Here's the drawing with two shaded views (mm, measured from the low corner). I have some questions. A direction names the side the tool comes from. Give positions to 0.01 mm unless a question says otherwise; leave off trailing zeros. Order: outer loops, then holes, each group sorted by start corner. A loop starts at its lowest first (then second) coordinate and runs counter-clockwise, first axis right, second up. Notation, with made-up numbers: M 34,63.25 L 73,63.25 A29 cw 73,84.25 Z; hole C 79.25,70 d6. An arc over 180 degrees is marked long. Use a Markdown table: item, result. Add a question column.
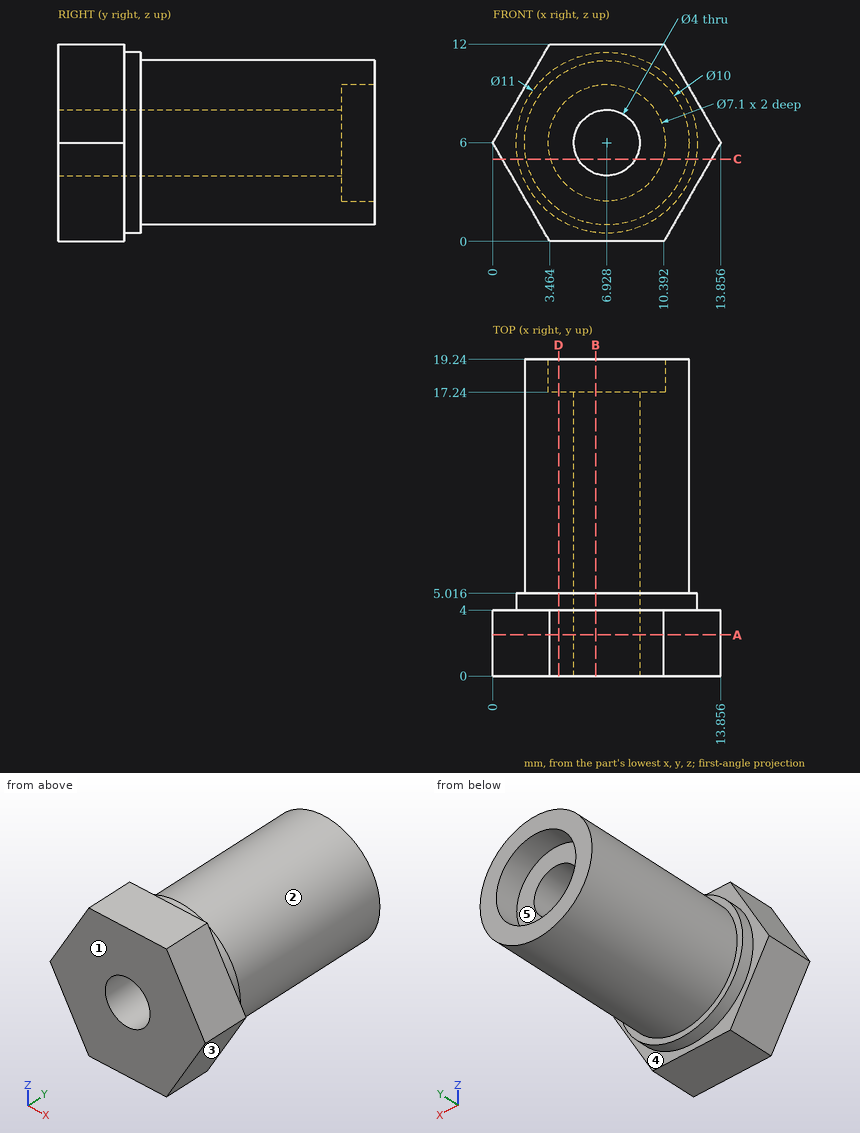
1) Suppose I cut it at A-A on y = 2.5. Please give me the cut outline in (x, z), and give its area (3 significant figures).
2) Suppose I cut it at C-C on z = 5. Please give me the cut outline in (x, y) (1 decimal), and give its area (3 significant figures).
3) For the marked faces 1 and 2, which set-ups out of +Z, -Z, +X, -X, +Y, -Y let a thin tool reach every point of the face, with its end or its side?
4) Please list where these lines run through material, in increasing order: line 1 (Y direction, x = 2.5, z = 3.5); line 2 (X direction, y = 10.25, z = 7) (1 decimal); line 3 (Y direction, x = 4.75, z = 5). Write a range as from..to.
5) Suppose I cut it at B-B on x = 6.25. Please give me the cut outline in (y, z) (1 decimal).
6) For pin 1 (4 mm diameter, centred on y = 16, z = 4.5, fed in from -X); pin 2 (5.5 mm diameter, centred on x = 6.93, z = 6, fed in from +Y); pin 3 (4 mm diameter, centred on y = 11.5, z = 6, fed in from +X); pin 4 (3 mm diameter, centred on x = 6.93, z = 6, fed in from +Y), each with a flat end and sliding along its axis, tell me the tip position at first contact or that it passes through.
7) We'd pull the mould along Z, two halves only. Please class the marked faces 3, 4 and 5: pulls with the +Z half, pulls with the -Z half, needs draft (parallel to the pull), parting line crosses it, or undercut.
8) Suppose I cut it at D-D on x = 4. Please give me the cut outline in (y, z) (1 decimal), and give its area (3 significant figures).
Values found:
| question | item | result |
|---|---|---|
| 1 | outline | M 0,6 L 3.46,0 L 10.39,0 L 13.86,6 L 10.39,12 L 3.46,12 Z; hole C 6.93,6 d4 |
| 1 | area | 112 mm^2 |
| 2 | outline | M 0.6,0 L 5.2,0 L 5.2,17.2 L 3.5,17.2 L 3.5,19.2 L 2,19.2 L 2,5 L 1.5,5 L 1.5,4 L 0.6,4 Z; M 8.7,0 L 13.3,0 L 13.3,4 L 12.3,4 L 12.3,5 L 11.8,5 L 11.8,19.2 L 10.3,19.2 L 10.3,17.2 L 8.7,17.2 Z |
| 2 | area | 128 mm^2 |
| 3 | face 1 | +Z, -Z, +X, -X, -Y |
| 3 | face 2 | +Y |
| 4 | line 1 | y = 0..5.02 |
| 4 | line 2 | x = 2..5.2, 8.7..11.8 |
| 4 | line 3 | y = 0..17.24 |
| 5 | outline | M 0,0 L 4,0 L 4,0.5 L 5,0.5 L 5,1 L 19.2,1 L 19.2,2.5 L 17.2,2.5 L 17.2,4.1 L 0,4.1 Z; M 0,7.9 L 17.2,7.9 L 17.2,9.5 L 19.2,9.5 L 19.2,11 L 5,11 L 5,11.5 L 4,11.5 L 4,12 L 0,12 Z |
| 6 | pin 1 | stops at x = 1.93 |
| 6 | pin 2 | stops at y = 17.24 |
| 6 | pin 3 | stops at x = 11.93 |
| 6 | pin 4 | passes through |
| 7 | face 3 | pulls with the -Z half |
| 7 | face 4 | needs draft |
| 7 | face 5 | undercut |
| 8 | outline | M 0,0 L 4,0 L 4,1.3 L 5,1.3 L 5,1.9 L 19.2,1.9 L 19.2,4 L 17.2,4 L 17.2,8 L 19.2,8 L 19.2,10.1 L 5,10.1 L 5,10.7 L 4,10.7 L 4,12 L 0,12 Z |
| 8 | area | 165 mm^2 |
